Input: part model. Units: mm. Frame: model coordinates. A direction names the side the tool comes from. Give positions to 0.01 mm unless a question says otherwise; leave off trailing zeros. Write each loop counter-clockwise with the first axis right and the second up, starting at its lowest first coordinate (ties: lowest second). Pieces come first, ordered by that corner, then holes. Notation, with made-up numbers: (8.5, 88.5) - (40.5, 88.5) arc R24 cw to (40.5, 108.5) - close; hole circle Ø9 at (19.5, 78). An arc over 180 degrees is marked (long way). Use a Markdown table: item, result. Add a question column.
1. Set-up query: faces 1 (the cylindrical face through (40, -1.5, 4.3)), 2 (the cylindrical face through (-14.58, -1.49, 8.42)), 3 (the flat face through (13.455, 0.74, 9.776)), 4 (the flat face through (-11.7, -4, -9)), 5 (the flat face through (15.31, 0.74, 10.54)). Return all of +Z, -Z, +X, -X, +Y, -Y with unobstructed straight access to the full face (end or side cutting, diameter ignored); none if empty.
2. Mould query, pull axis Z, two halves, no side actions, for faces 6 (the cylindrical face through (-14.44, 2.49, 11.98)), 7 (the flat face through (0, -5, 17)), 8 (the cylindrical face through (3.763, -24.479, 10.402)), 9 (the flat face through (26, -1, 5)). Classes: released by +Z, released by -Z, zero draft, split by the parting line, or undercut.
3. Section query B-B, the plane y = -17.5. Return loops of the section in (x, z).
4. Section query D-D, the plane x = -27. Return loops of the section in (y, z), plus the area to 3 significant figures.
5. Pin query (flat end, axial travel): pin 1 (0.8 mm diameter, centred on y = -0.5, z = -1.5, fed in from +X); pin 2 (1.5 mm diameter, centred on x = 21, z = 4.5, fed in from +Y); pin 3 (0.5 mm diameter, centred on x = 24.5, y = -1.5, fed in from +Z). Return the tip coordinate at first contact, or that it passes through.
6. Section query C-C, the plane z = 15.5. Return loops of the section in (x, y).
7. Section query A-A, the plane x = 0. Return loops of the section in (y, z).
8. Material intervals for probe 1 along Z at (x, y) = (-30, -15.4); probe 2 along Z at (x, y) = (17.5, -10.65); probe 3 along Z at (x, y) = (-23, -10.75), sorted ascending.
```python
from build123d import *

# Parameters (mm, degrees)
F0_W      = 32
F0_H      = 26
F1_DEPTH  = 1
F3_DEPTH  = 1
F4_R      = 9
F4_R_2    = 8
F5_DEPTH  = 14
F6_R      = 2.5
F6_R_2    = 1.5
F7_DEPTH  = 9
F8_W      = 22
F8_H      = 5
F9_DEPTH  = 2.5
F10_W     = 16
F10_H     = 16.5
F11_DEPTH = 3
F13_DEPTH = 3
F14_R     = 7
F15_DEPTH = 6
F16_R     = 5.5
F17_DEPTH = 10
F18_R     = 7
F19_DEPTH = 3
F20_DEPTH = 13
F21_DEPTH = 8
F22_R     = 1.2
F23_DEPTH = 1
F24_R     = 0.5
F26_DEPTH = 1.5
F27_R     = 0.75
F28_DEPTH = 2
F29_W     = 4
F29_H     = 7
F30_DEPTH = 6
F31_R     = 0.25
F32_DEPTH = 2
F33_R     = 0.25
F34_DEPTH = 1


with BuildPart() as f1:
    # F0 (on Front) → F1 (new body)
    with BuildSketch(Plane.XZ):
        Rectangle(F0_W, F0_H)
    extrude(amount=F1_DEPTH)

    # F2 (on face) → F3 (join)
    with BuildSketch(Plane.XZ.offset(1)):
        with BuildLine():
            ThreePointArc((-13.3333333333, 10.1366100188), (-12.6645691026, 12.8920552244), (-15, 14.5))
            Line((-15, 14.5), (-30, 14.5))
            ThreePointArc((-30, 14.5), (-40, 4.5), (-30, -5.5))
            Line((-30, -5.5), (-15, -5.5))
            ThreePointArc((-15, -5.5), (-12.6645691026, -3.8920552244), (-13.3333333333, -1.1366100188))
            ThreePointArc((-13.3333333333, -1.1366100188), (-14.5643546459, 0.5489284914), (-15, 2.5901699437))
            Line((-15, 2.5901699437), (-15, 6.4098300563))
            ThreePointArc((-15, 6.4098300563), (-14.5643546459, 8.4510715086), (-13.3333333333, 10.1366100188))
        make_face()
        with BuildLine():
            ThreePointArc((13.3333333333, 10.1366100188), (14.5643546459, 8.4510715086), (15, 6.4098300563))
            Line((15, 6.4098300563), (15, 2.5901699437))
            ThreePointArc((15, 2.5901699437), (14.5643546459, 0.5489284914), (13.3333333333, -1.1366100188))
            ThreePointArc((13.3333333333, -1.1366100188), (12.6645691026, -3.8920552244), (15, -5.5))
            Line((15, -5.5), (30, -5.5))
            ThreePointArc((30, -5.5), (40, 4.5), (30, 14.5))
            Line((30, 14.5), (15, 14.5))
            ThreePointArc((15, 14.5), (12.6645691026, 12.8920552244), (13.3333333333, 10.1366100188))
        make_face()
    extrude(amount=F3_DEPTH)

    # F4 (on face) → F5 (join)
    with BuildSketch(Plane.XZ.offset(2)):
        with Locations((-30, 4.5)):
            Circle(F4_R)
        with Locations((-30, 4.5)):
            Circle(F4_R_2, mode=Mode.SUBTRACT)
        with Locations((30, 4.5)):
            Circle(F4_R)
        with Locations((30, 4.5)):
            Circle(F4_R_2, mode=Mode.SUBTRACT)
    extrude(amount=F5_DEPTH)

    # F6 (on face) → F7 (join)
    with BuildSketch(Plane.XZ.offset(2)):
        with Locations((-17.5, 12)):
            Circle(F6_R)
        with Locations((-17.5, 12)):
            Circle(F6_R_2, mode=Mode.SUBTRACT)
        with Locations((17.5, -3)):
            Circle(F6_R)
        with Locations((17.5, -3)):
            Circle(F6_R_2, mode=Mode.SUBTRACT)
    extrude(amount=F7_DEPTH)

    # F8 (on face) → F9 (join)
    with BuildSketch(Plane.XZ.offset(1)):
        with Locations((0, -10)):
            Rectangle(F8_W, F8_H)
    extrude(amount=F9_DEPTH)

    # F10 (on face) → F11 (join)
    with BuildSketch(Plane.XZ.offset(1)):
        with Locations((0, 4.75)):
            Rectangle(F10_W, F10_H)
    extrude(amount=F11_DEPTH)

    # F12 (on face) → F13 (join)
    with BuildSketch(Plane.XZ.offset(4)):
        with BuildLine():
            Line((5, 17), (-5, 17))
            ThreePointArc((-5, 17), (-10.0070053709, 14.2599828397), (-12, 8.9115466915))
            Line((-12, 8.9115466915), (-12, 0))
            ThreePointArc((-12, 0), (-10.170162501, -5.153882032), (-5.5, -8))
            Line((-5.5, -8), (5.5, -8))
            ThreePointArc((5.5, -8), (10.170162501, -5.153882032), (12, 0))
            Line((12, 0), (12, 8.9115466915))
            ThreePointArc((12, 8.9115466915), (10.0070053709, 14.2599828397), (5, 17))
        make_face()
    extrude(amount=F13_DEPTH)

    # F14 (on face) → F15 (join)
    with BuildSketch(Plane.XZ.offset(7)):
        with Locations((0, 4.5)):
            Circle(F14_R)
    extrude(amount=F15_DEPTH)

    # F16 (on face) → F17 (join)
    with BuildSketch(Plane.XZ.offset(13)):
        with Locations((0, 4.5)):
            Circle(F16_R)
    extrude(amount=F17_DEPTH)

    # F18 (on face) → F19 (join)
    with BuildSketch(Plane.XZ.offset(23)):
        with Locations((0, 4.5)):
            Circle(F18_R)
    extrude(amount=F19_DEPTH)

    # F20 (add): faces of the model
    f20_faces = [f1.faces().sort_by_distance(p)[0] for p in [
        (-30, -2, 4.5),
        (30, -2, 4.5),
    ]]
    extrude(f20_faces, amount=F20_DEPTH)

    # F21 (add): faces of the model
    f21_faces = [f1.faces().sort_by_distance(p)[0] for p in [
        (17.5, -2, -3),
        (-17.5, -2, 12),
    ]]
    extrude(f21_faces, amount=F21_DEPTH)

    # F22 (on face) → F23 (join)
    with BuildSketch(Plane.XZ.offset(2)):
        with Locations((-13.7226518032, 11.7583771864)):
            Circle(F22_R)
        with Locations((-13.7226518032, -3.2416228136)):
            Circle(F22_R)
        with Locations((13.7226518032, 11.7583771864)):
            Circle(F22_R)
        with Locations((13.7226518032, -3.2416228136)):
            Circle(F22_R)
    extrude(amount=F23_DEPTH)

    # F24
    f24_edges = [f1.edges().sort_by_distance(p)[0] for p in [
        (-14.922652, -3, 11.758377),
        (-14.922652, -3, -3.241623),
        (12.522652, -3, 11.758377),
        (12.522652, -3, -3.241623),
    ]]
    fillet(f24_edges, radius=F24_R)

    # F25 (on face) → F26 (join)
    with BuildSketch(Plane(origin=(0, 0, 0), x_dir=(-1, 0, 0), z_dir=(0, 1, 0))):
        Polygon((-15.1497724348, 13.5740478713), (-16.008629057, 11.4302898075), (-14.5815084254, 9.6146191226), (-12.2955311715, 9.9427065015), (-11.4366745493, 12.0864645652), (-12.863795181, 13.9021352501), align=None)
        Polygon((15.3299889793, 10.1001249331), (15.9624089685, 12.3212458867), (14.3550717923, 13.97949814), (12.115314627, 13.4166294396), (11.4828946379, 11.195508486), (13.090231814, 9.5372562327), align=None)
        Polygon((-13.2535514476, -5.5028787014), (-11.5297965822, -3.9659979326), (-11.9988969377, -1.7047420449), (-14.1917521587, -0.9803669259), (-15.9155070242, -2.5172476946), (-15.4464066686, -4.7785035823), align=None)
        Polygon((13.9503915154, -5.5397672732), (15.8267731428, -4.1934666672), (15.5990334306, -1.8953222076), (13.494912091, -0.9434783541), (11.6185304636, -2.2897789601), (11.8462701758, -4.5879234196), align=None)
    extrude(amount=F26_DEPTH)

    # F27 (on face) → F28 (join)
    with BuildSketch(Plane(origin=(0, 1.5, 0), x_dir=(-1, 0, 0), z_dir=(0, 1, 0))):
        with Locations((-13.7226518032, 11.7583771864)):
            Circle(F27_R)
        with Locations((-13.7226518032, -3.2416228136)):
            Circle(F27_R)
        with Locations((13.7226518032, -3.2416228136)):
            Circle(F27_R)
        with Locations((13.7226518032, 11.7583771864)):
            Circle(F27_R)
    extrude(amount=F28_DEPTH)

    # F29 (on face) → F30 (join)
    with BuildSketch(Plane.XZ.offset(1)):
        with Locations((-13.7, -9.2)):
            Rectangle(F29_W, F29_H)
    extrude(amount=F30_DEPTH)

    # F31 (on face) → F32 (join)
    with BuildSketch(Plane(origin=(-12, 0, 0), x_dir=(0, -1, 0), z_dir=(-1, 0, 0))):
        with Locations((5.5, 12.1115466915)):
            Circle(F31_R)
        with Locations((5.5, 11.4115466915)):
            Circle(F31_R)
    extrude(amount=-F32_DEPTH)

    # F33 (on face) → F34 (join)
    with BuildSketch(Plane.XZ.offset(7)):
        with Locations((-13.7, -8.85)):
            Circle(F33_R)
        with Locations((-13.7, -9.55)):
            Circle(F33_R)
    extrude(amount=F34_DEPTH)


solid = f1.part
```
Result sheet:
| question | item | result |
|---|---|---|
| 1 | face 1 | +X, +Y, -Y |
| 1 | face 2 | -Y |
| 1 | face 3 | +Y |
| 1 | face 4 | -Z, -Y |
| 1 | face 5 | +X, +Y |
| 2 | face 6 | undercut |
| 2 | face 7 | released by +Z |
| 2 | face 8 | split by the parting line |
| 2 | face 9 | zero draft |
| 3 | outline | circle Ø11 at (0, 4.5) |
| 4 | outline | (-16, -3.99) - (-2, -3.99) - (-2, -5.5) - (-1, -5.5) - (-1, 14.5) - (-2, 14.5) - (-2, 12.99) - (-16, 12.99) - (-16, 11.92) - (-15, 11.92) - (-15, -2.92) - (-16, -2.92) - close |
| 4 | area | 243 mm² |
| 5 | pin 1 | stops at x = 16 |
| 5 | pin 2 | stops at y = -1 |
| 5 | pin 3 | stops at z = 14.5 |
| 6 | outline | (-8.66, -7) - (8.66, -7) - (8.66, -4) - (-8.66, -4) - close |
| 7 | outline | (-26, -2.5) - (-23, -2.5) - (-23, -1) - (-13, -1) - (-13, -2.5) - (-7, -2.5) - (-7, -8) - (-4, -8) - (-4, -3.5) - (-1, -3.5) - (-1, -7.5) - (-3.5, -7.5) - (-3.5, -12.5) - (-1, -12.5) - (-1, -13) - (0, -13) - (0, 13) - (-4, 13) - (-4, 17) - (-7, 17) - (-7, 11.5) - (-13, 11.5) - (-13, 10) - (-23, 10) - (-23, 11.5) - (-26, 11.5) - close |
| 8 | probe 1 | z = -4.5 to -3.5, 12.5 to 13.5 |
| 8 | probe 2 | z = -5.5 to -4.5, -1.5 to -0.5 |
| 8 | probe 3 | z = -1.16 to 10.16 |
